Part model, mm, in its own coordinate system. A direction names the side the tool comes from. Coordinates: 2 decimals unless noted, no trailing zeros. Loops run counter-clockwise (first coordinate to the right, second up) from the corner with the lowest first, then second, coordinate; pieces in that order, holes last. Notation, with made-up numbers: M 87,38 L 119,38 A11 ccw 119,45 Z; hole C 59.5,-6 d7. An arc over 180 degrees is marked long. Answer as CSV lines item,"result". Start each with the question number.
from build123d import *

# Parameters (mm, degrees)
RESSALTO_EXTRUS_O1_DEPTH = 1.4
ESBO_O2_R                = 3.45
RESSALTO_EXTRUS_O2_DEPTH = 2.4
FURO1_D                  = 1.2
PADR_O_LINEAR1_COUNT     = 6
PADR_O_LINEAR1_PITCH     = 2
RESSALTO_EXTRUS_O3_DEPTH = 1.4
FURO2_D                  = 1.2
PADR_O_LINEAR2_COUNT     = 7
PADR_O_LINEAR2_PITCH     = 2
RESSALTO_EXTRUS_O4_DEPTH = 1.4
FURO3_D                  = 1.2
PADR_O_LINEAR3_COUNT     = 2
PADR_O_LINEAR3_PITCH     = 2
PADR_OCIRCULAR1_COUNT    = 2
PADR_OCIRCULAR1_COPY_1_D = 1.2
FURO4_D                  = 4.95
FURO4_DEPTH              = 2
FURO5_D                  = 4.6
FURO5_DEPTH              = 1
FURO6_D                  = 2.1
RESSALTO_EXTRUS_O5_START = -2
RESSALTO_EXTRUS_O5_DEPTH = 2
PADR_OCIRCULAR2_COUNT    = 60
BOSS_EXTRUDE1_DEPTH      = 5
BOSS_EXTRUDE1_2_DEPTH    = 5
BOSS_EXTRUDE1_3_DEPTH    = 5
SKETCH2_W                = 100
SKETCH2_H                = 17.359649926
BOSS_EXTRUDE2_DEPTH      = 2.5
SKETCH3_R                = 1.3
CUT_EXTRUDE1_DEPTH       = 92.764859077
SKETCH4_W                = 52.17150673
SKETCH4_H                = 37.712890546
CUT_EXTRUDE2_DEPTH       = 92.649055431
CUT_EXTRUDE3_DEPTH       = 2.5
SKETCH6_W                = 5
SKETCH6_H                = 17.359649926
CUT_EXTRUDE5_DEPTH       = 10


with BuildPart() as part:
    # Esboço1 → Ressalto-extrusão1 (new body)
    with BuildSketch(Plane(origin=(0, 0, 0), x_dir=(1, 0, 0), z_dir=(0, 1, 0))):
        with BuildLine():
            Line((-14.159121967, 1.99702088), (-2.209072203, 2.65))
            ThreePointArc((-2.209072203, 2.65), (3.45, 0), (-2.209072203, -2.65))
            Line((-2.209072203, -2.65), (-14.159121967, -1.99702088))
            ThreePointArc((-14.159121967, -1.99702088), (-16.05, 0), (-14.159121967, 1.99702088))
        make_face()
    extrude(amount=-RESSALTO_EXTRUS_O1_DEPTH)

    # Esboço2 → Ressalto-extrusão2 (add)
    with BuildSketch(Plane.XZ.offset(1.4)):
        with Locations(Location((0, 0, 0), (0, 0, 90))):
            Circle(ESBO_O2_R)
    extrude(amount=RESSALTO_EXTRUS_O2_DEPTH)

    # Furo1 (through all)
    with Locations(Plane(origin=(0, 0, 0), x_dir=(1, 0, 0), z_dir=(0, 1, 0))):
        with Locations((-14.45, 0)):
            furo1 = Hole(FURO1_D / 2)

    # Padrão linear1: Furo1 ×6
    with Locations(*[(i * PADR_O_LINEAR1_PITCH, 0, 0) for i in range(1, PADR_O_LINEAR1_COUNT)]):
        add(furo1, mode=Mode.SUBTRACT)

    # Esboço12 → Ressalto-extrusão3 (add)
    with BuildSketch(Plane(origin=(0, 0, 0), x_dir=(1, 0, 0), z_dir=(0, 1, 0))):
        with BuildLine():
            Line((0.304103343, 3.436571134), (16.626291793, 1.99221515))
            ThreePointArc((16.626291793, 1.99221515), (18.45, 0), (16.626291793, -1.99221515))
            Line((16.626291793, -1.99221515), (0.304103343, -3.436571134))
            ThreePointArc((0.304103343, -3.436571134), (3.45, 0), (0.304103343, 3.436571134))
        make_face()
    extrude(amount=-RESSALTO_EXTRUS_O3_DEPTH)

    # Furo2 (through all)
    with Locations(Plane(origin=(0, 0, 0), x_dir=(1, 0, 0), z_dir=(0, 1, 0))):
        with Locations((16.85, 0)):
            furo2 = Hole(FURO2_D / 2)

    # Padrão linear2: Furo2 ×7
    with Locations(*[(-i * PADR_O_LINEAR2_PITCH, 0, 0) for i in range(1, PADR_O_LINEAR2_COUNT)]):
        add(furo2, mode=Mode.SUBTRACT)

    # Esboço16 → Ressalto-extrusão4 (add)
    with BuildSketch(Plane(origin=(0, 0, 0), x_dir=(1, 0, 0), z_dir=(0, 1, 0))):
        with BuildLine():
            Line((-1.9, -6.45), (-1.9, 6.45))
            ThreePointArc((-1.9, 6.45), (0, 8.35), (1.9, 6.45))
            Line((1.9, 6.45), (1.9, -6.45))
            ThreePointArc((1.9, -6.45), (0, -8.35), (-1.9, -6.45))
        make_face()
    extrude(amount=-RESSALTO_EXTRUS_O4_DEPTH)

    # Furo3 (through all)
    with Locations(Plane(origin=(0, 0, 0), x_dir=(1, 0, 0), z_dir=(0, 1, 0))):
        with Locations((0, -6.45)):
            furo3 = Hole(FURO3_D / 2)

    # Padrão linear3: Furo3 ×2
    with Locations(*[(0, 0, -i * PADR_O_LINEAR3_PITCH) for i in range(1, PADR_O_LINEAR3_COUNT)]):
        add(furo3, mode=Mode.SUBTRACT)

    # PadrãoCircular1: Furo3 ×2 about axis
    padr_ocircular1_axis = Axis((0, 0, 0), (0, 1, 0))
    for i in range(1, PADR_OCIRCULAR1_COUNT):
        add(furo3.rotate(padr_ocircular1_axis, i * 360 / PADR_OCIRCULAR1_COUNT), mode=Mode.SUBTRACT)

    # PadrãoCircular1 copy 1 (through all)
    with Locations(Plane(origin=(0, 0, 2), x_dir=(-1, 0, 0), z_dir=(0, 1, 0))):
        with Locations((0, -6.45)):
            Hole(PADR_OCIRCULAR1_COPY_1_D / 2)

    # Furo4
    with Locations(Plane(origin=(0, -3.8, 0), x_dir=(-1, 0, 0), z_dir=(0, -1, 0))):
        with Locations((0, 0)):
            Hole(FURO4_D / 2, depth=FURO4_DEPTH)

    # Furo5
    with Locations(Plane(origin=(0, 0, 0), x_dir=(1, 0, 0), z_dir=(0, 1, 0))):
        with Locations((0, 0)):
            Hole(FURO5_D / 2, depth=FURO5_DEPTH)

    # Furo6 (through all)
    with Locations(Plane(origin=(0, 0, 0), x_dir=(1, 0, 0), z_dir=(0, 1, 0))):
        with Locations((0, 0)):
            Hole(FURO6_D / 2)

    # Esboço11 → Ressalto-extrusão5 (add)
    with BuildSketch(Plane.XZ.offset(3.8).offset(RESSALTO_EXTRUS_O5_START)):
        with BuildLine():
            Line((-0.098056786, 2.473056786), (0, 2.375))
            Line((0, 2.375), (0.098056786, 2.473056786))
            ThreePointArc((0.098056786, 2.473056786), (0, 2.475), (-0.098056786, 2.473056786))
        make_face()
    ressalto_extrus_o5 = extrude(amount=RESSALTO_EXTRUS_O5_DEPTH)

    # PadrãoCircular2: Ressalto-extrusão5 ×60 about axis
    padr_ocircular2_axis = Axis((0, 0, 0), (0, 1, 0))
    for i in range(1, PADR_OCIRCULAR2_COUNT):
        add(ressalto_extrus_o5.rotate(padr_ocircular2_axis, i * 360 / PADR_OCIRCULAR2_COUNT))


with BuildPart() as body_2:
    # Sketch1 → Boss-Extrude1 (new body)
    with BuildSketch(Plane(origin=(0, 0, 0), x_dir=(1, 0, 0), z_dir=(0, 1, 0))):
        with BuildLine():
            ThreePointArc((-2.9, 6.45), (-2.625551521, 7.681454104), (-1.854152269, 8.679824963))
            Line((-1.854152269, 8.679824963), (-91.1, 8.679824963))
            Line((-91.1, 8.679824963), (-91.1, -8.679824963))
            Line((-91.1, -8.679824963), (-1.854152269, -8.679824963))
            ThreePointArc((-1.854152269, -8.679824963), (-2.625551521, -7.681454104), (-2.9, -6.45))
            Line((-2.9, -6.45), (-2.9, -3.613737845))
            Line((-2.9, -3.613737845), (-14.213682951, -2.99553132))
            ThreePointArc((-14.213682951, -2.99553132), (-17.05, 0), (-14.213682951, 2.99553132))
            Line((-14.213682951, 2.99553132), (-2.9, 3.613737845))
            Line((-2.9, 3.613737845), (-2.9, 6.45))
        make_face()
    extrude(amount=BOSS_EXTRUDE1_DEPTH)



with BuildPart() as body_3:
    # Sketch1 → Boss-Extrude1 2 (new body)
    with BuildSketch(Plane(origin=(0, 0, 0), x_dir=(1, 0, 0), z_dir=(0, 1, 0))):
        with BuildLine():
            Line((2.9, 4.210766995), (8.9, 3.679824963))
            Line((8.9, 3.679824963), (8.9, 8.679824963))
            Line((8.9, 8.679824963), (1.854152269, 8.679824963))
            ThreePointArc((1.854152269, 8.679824963), (2.625551521, 7.681454104), (2.9, 6.45))
            Line((2.9, 6.45), (2.9, 4.210766995))
        make_face()
    extrude(amount=BOSS_EXTRUDE1_2_DEPTH)


with BuildPart() as body_4:
    # Sketch1 → Boss-Extrude1 3 (new body)
    with BuildSketch(Plane(origin=(0, 0, 0), x_dir=(1, 0, 0), z_dir=(0, 1, 0))):
        with BuildLine():
            Line((8.9, -8.679824963), (8.9, -3.679824963))
            Line((8.9, -3.679824963), (2.9, -4.210766995))
            Line((2.9, -4.210766995), (2.9, -6.45))
            ThreePointArc((2.9, -6.45), (2.625551521, -7.681454104), (1.854152269, -8.679824963))
            Line((1.854152269, -8.679824963), (8.9, -8.679824963))
        make_face()
    extrude(amount=BOSS_EXTRUDE1_3_DEPTH)


with BuildPart() as body_2_1:
    add(body_2.part)

    add(body_3.part)  # Boss-Extrude2 merges body 3

    add(body_4.part)  # Boss-Extrude2 merges body 4
    # Sketch2 → Boss-Extrude2 (add)
    with BuildSketch(Plane(origin=(0, 5, 0), x_dir=(1, 0, 0), z_dir=(0, 1, 0))):
        with Locations((-41.1, 0)):
            Rectangle(SKETCH2_W, SKETCH2_H)
    extrude(amount=-BOSS_EXTRUDE2_DEPTH)


with BuildPart() as cut_extrude1_tool:
    # Sketch3 → Cut-Extrude1 (new, through all)
    with BuildSketch(Plane.XZ.offset(1.8)):
        with Locations(Location((0, 0, 0), (0, 0, 270))):
            Circle(SKETCH3_R)
    extrude(amount=-CUT_EXTRUDE1_DEPTH)


with BuildPart() as part_1:
    add(part.part)

    # Cut-Extrude1: cut by cut_extrude1_tool
    add(cut_extrude1_tool.part, mode=Mode.SUBTRACT)

    # Sketch4 → Cut-Extrude2 (cut, through all)
    with BuildSketch(Plane.XZ):
        with Locations((5.123033061, -1.807327023)):
            Rectangle(SKETCH4_W, SKETCH4_H)
    extrude(amount=CUT_EXTRUDE2_DEPTH, mode=Mode.SUBTRACT)


with BuildPart() as body_2_2:
    add(body_2_1.part)

    # Cut-Extrude1: cut by cut_extrude1_tool
    add(cut_extrude1_tool.part, mode=Mode.SUBTRACT)

    # Sketch5 → Cut-Extrude3 (cut)
    with BuildSketch(Plane.XZ):
        with BuildLine():
            Line((-14.213682951, 2.99553132), (-21.713682951, 2.585713496))
            ThreePointArc((-21.713682951, 2.585713496), (-24.299396446, 0), (-21.713682951, -2.585713496))
            Line((-21.713682951, -2.585713496), (-14.213682951, -2.99553132))
            Line((-14.213682951, -2.99553132), (-14.213682951, 2.99553132))
        make_face()
    extrude(amount=-CUT_EXTRUDE3_DEPTH, mode=Mode.SUBTRACT)

    # Sketch6 → Cut-Extrude5 (cut)
    with BuildSketch(Plane.XZ):
        with Locations((6.4, 0)):
            Rectangle(SKETCH6_W, SKETCH6_H)
    extrude(amount=-CUT_EXTRUDE5_DEPTH, mode=Mode.SUBTRACT)


solid = body_2_2.part
Q1. Slice it at C-C, the plane z = -5.25. Write the cut outline in (x, y), and give its area (4 significant figures).
Q2. Wall check: L1, parallel to X at y = 0.8, z = 6.5; L2, parallel to X at y = 3.55, z = 0; L3, parallel to Z at x = -22.5, y = 1.1. Give the ranges that are in metal, low to high.
Q3. Tool access for faces 1 (the face through (-7, 2.5, 0)), 2 (the face through (-44, 5, 0)): list every direction of +Z, -Z, +X, -X, +Y, -Y with a clear straight run to the whole face (end or side of a thin tool).
Q4. Slice it at A-A, the plane z = 0. Write the cut outline in (x, y), and give its area (3 significant figures).
Q5. Two-plate mould, pull along X, no slides. Class faces 3 (the face through (-2.618, 1.232, 7.698)), 4 (the face through (-43, 2, -8.68)), 5 (the face through (-24.3, 1.23, 0.06)): +X half, -X half, draft (parallel to the pull), parting line (faces both ways), or undercut.
Q6. Slice it at B-B, the plane x = 0. Write the cut outline in (y, z), and give its area (3 significant figures).
Q7. Flat gauge pin, fed straight in: P1, Ø3, axis at x = 0, z = 0, coming from the -Y side. Where does the tip first touch, or does it go through?
Solved:
1,outline,"M -91.1,0 L -2.9,0 L -2.9,2.5 L 2.9,2.5 L 2.9,0 L 3.9,0 L 3.9,5 L -91.1,5 Z"
1,area,"460.5 mm2"
2,L1,"x = -91.1 to -2.9, 2.9 to 3.9"
2,L2,"x = -91.1 to -1.3, 1.3 to 3.9"
2,L3,"z = -8.68 to -2.46, 2.46 to 8.68"
3,face 1,"-Y"
3,face 2,"+Z, -Z, +X, -X, +Y"
4,outline,"M -91.1,0 L -24.3,0 L -24.3,2.5 L -1.3,2.5 L -1.3,5 L -91.1,5 Z; M 1.3,2.5 L 3.9,2.5 L 3.9,5 L 1.3,5 Z"
4,area,"398 mm2"
5,face 3,"undercut"
5,face 4,"draft"
5,face 5,"+X half"
6,outline,"M 2.5,-8.68 L 5,-8.68 L 5,-1.3 L 2.5,-1.3 Z; M 2.5,1.3 L 5,1.3 L 5,8.68 L 2.5,8.68 Z"
6,area,"36.9 mm2"
7,P1,"stops at y = 2.5"
